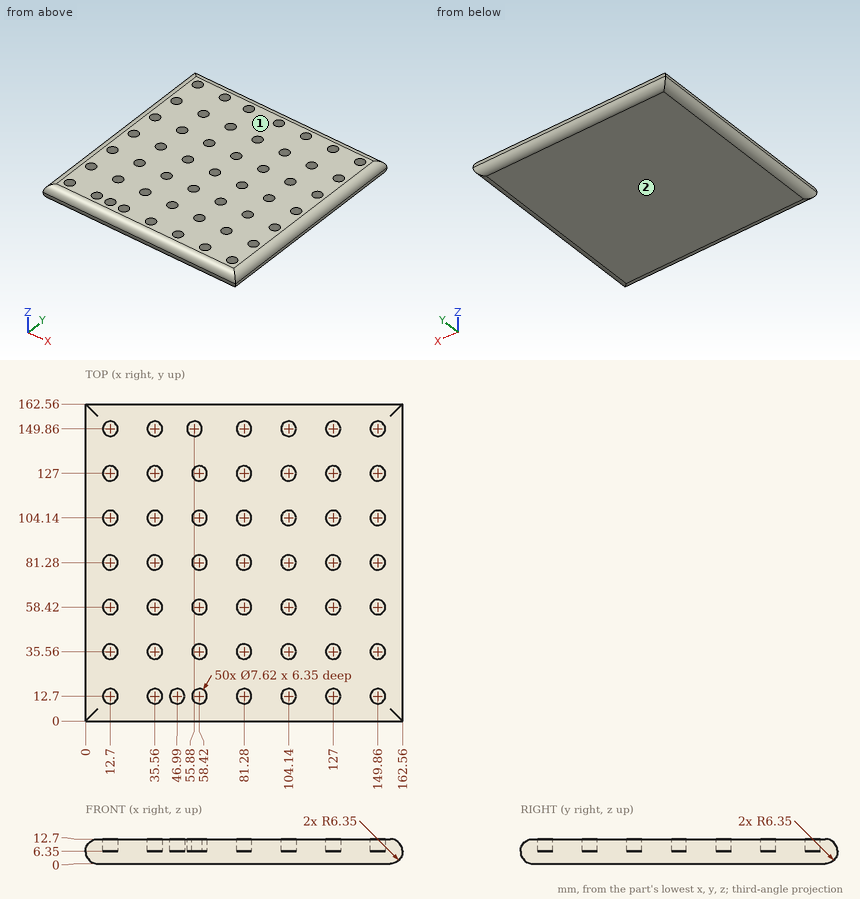
Geometry: see drawing. Coordinates: mm, zero at the bounding-box minimum. Round coordinates to 2 decimals unless told otherwise and drop trailing zeros. Use a Markdown table: item, result. Add a question column.
1. Ray query, line 1 along Y through (x, z) = (46.99, 8.5); line 2 along Y through (x, z) = (77, 7); line 3 along Y through (x, z) = (45.5, 4). Return the intervals inside material, ascending. Write a range as [from, to].
2. Contact query for flat-ended pins moving along their axis: pin 1 (1 mm diameter, centred on x = 115.5, y = 84.5, fed in from -Z); pin 2 (6 mm diameter, centred on x = 58.42, y = 81.28, fed in from +Z); pin 3 (1 mm diameter, centred on x = 104.5, z = 8, fed in from -Y) (3 decimals); pin 4 (4 mm diameter, centred on x = 79, z = 4, fed in from -Y). Output: stop coordinate, or through.
3. Pull-direction query (Z, two-part tool) for the marked faces 1 and 2; classes: +Z half, -Z half, draft (parallel to the pull), parting line (faces both ways), or undercut.
Solution:
| question | item | result |
|---|---|---|
| 1 | line 1 | y = [0.38, 8.89], [16.51, 162.18] |
| 1 | line 2 | y = [0.03, 162.53] |
| 1 | line 3 | y = [0.45, 162.11] |
| 2 | pin 1 | stops at z = 0 |
| 2 | pin 2 | stops at z = 6.35 |
| 2 | pin 3 | stops at y = 0.105 |
| 2 | pin 4 | stops at y = 0.01 |
| 3 | face 1 | +Z half |
| 3 | face 2 | -Z half |
